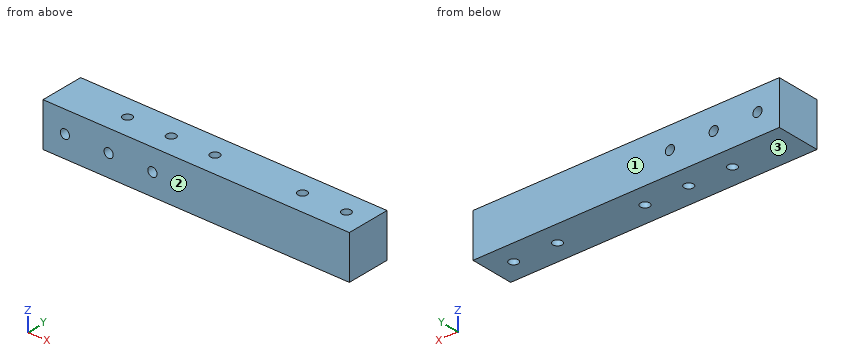
from build123d import *

# Parameters (mm, degrees)
SKETCH_1_W          = 20
SKETCH_1_H          = 20
EXTRUDE_1_DEPTH     = 140
SKETCH_3_R          = 2.1
CUT_EXTRUDE_1_DEPTH = 142.774468788
SKETCH_2_R          = 2.1
CUT_EXTRUDE_2_DEPTH = 142.774468788


with BuildPart() as part:
    # 草图1 → 凸台-拉伸1 (new body)
    with BuildSketch(Plane(origin=(0, 0, 0), x_dir=(0, 0, -1), z_dir=(1, 0, 0))):
        Rectangle(SKETCH_1_W, SKETCH_1_H)
    extrude(amount=EXTRUDE_1_DEPTH)

    # 草图3 → 切除-拉伸1 (cut, through all)
    with BuildSketch(Plane.XY.offset(10)):
        with Locations((30, 0)):
            Circle(SKETCH_3_R)
        with Locations((50, 0)):
            Circle(SKETCH_3_R)
        with Locations((70, 0)):
            Circle(SKETCH_3_R)
        with Locations((130, 0)):
            Circle(SKETCH_3_R)
        with Locations((110, 0)):
            Circle(SKETCH_3_R)
    extrude(amount=-CUT_EXTRUDE_1_DEPTH, mode=Mode.SUBTRACT)

    # 草图2 → 切除-拉伸2 (cut, through all)
    with BuildSketch(Plane(origin=(0, 10, 0), x_dir=(1, 0, 0), z_dir=(0, 1, 0))):
        with Locations(Location((10, 0, 0), (0, 0, 270))):
            Circle(SKETCH_2_R)
        with Locations(Location((30, 0, 0), (0, 0, 270))):
            Circle(SKETCH_2_R)
        with Locations(Location((50, 0, 0), (0, 0, 270))):
            Circle(SKETCH_2_R)
    extrude(amount=-CUT_EXTRUDE_2_DEPTH, mode=Mode.SUBTRACT)


solid = part.part
Check sheet for the modelled part. Datum: model origin and axes. Units: mm. Face numbers are marked on the shaded views. Give positions to 0.01 mm unless a question says otherwise; leave off trailing zeros. Loops run counter-clockwise (first coordinate to the right, second up) from the corner with the lowest first, then second, coordinate; pieces in that order, holes last. Notation, with made-up numbers: M 52.25,69.25 L 66.25,69.25 A32 ccw 66.25,97.25 Z; hole C 65.25,68 d2. An arc over 180 degrees is marked long. Answer as a JSON object with one key per item and string values. Group by question number.
Q1. Release check for a two-part mould opening along Y. For the marked faces 1, 2 and 3 record: released by +Y, released by -Y, zero draft, split by the parting line, or undercut.
Q2. Cross-section at B-B on x = 10. Record the cut outline in (y, z).
Q3. Material ranges on line 1 along X through (y, z) = (-2.25, 0); line 2 along X through (y, z) = (-2.25, -1.25); line 3 along Y through (x, z) = (110, 0.5), recorded low to high. Write a range as [from, to].
Q4. Cross-section at A-A on z = 8. Record the cut outline in (x, y), then the cut area to 3 significant figures.
Evaluation:
{
 "1": {"face 1": "released by +Y", "face 2": "released by -Y", "face 3": "zero draft"},
 "2": {"outline": "M -10,-10 L 10,-10 L 10,-2.1 L -10,-2.1 Z; M -10,2.1 L 10,2.1 L 10,10 L -10,10 Z"},
 "3": {"line 1": "x = [0, 7.9], [12.1, 27.9], [32.1, 47.9], [52.1, 140]", "line 2": "x = [0, 8.31], [11.69, 28.31], [31.69, 48.31], [51.69, 140]", "line 3": "y = [-10, -2.1], [2.1, 10]"},
 "4": {"outline": "M 0,-10 L 140,-10 L 140,10 L 0,10 Z; hole C 30,0 d4.2; hole C 50,0 d4.2; hole C 70,0 d4.2; hole C 110,0 d4.2; hole C 130,0 d4.2", "area": "2,730 mm2"}
}
